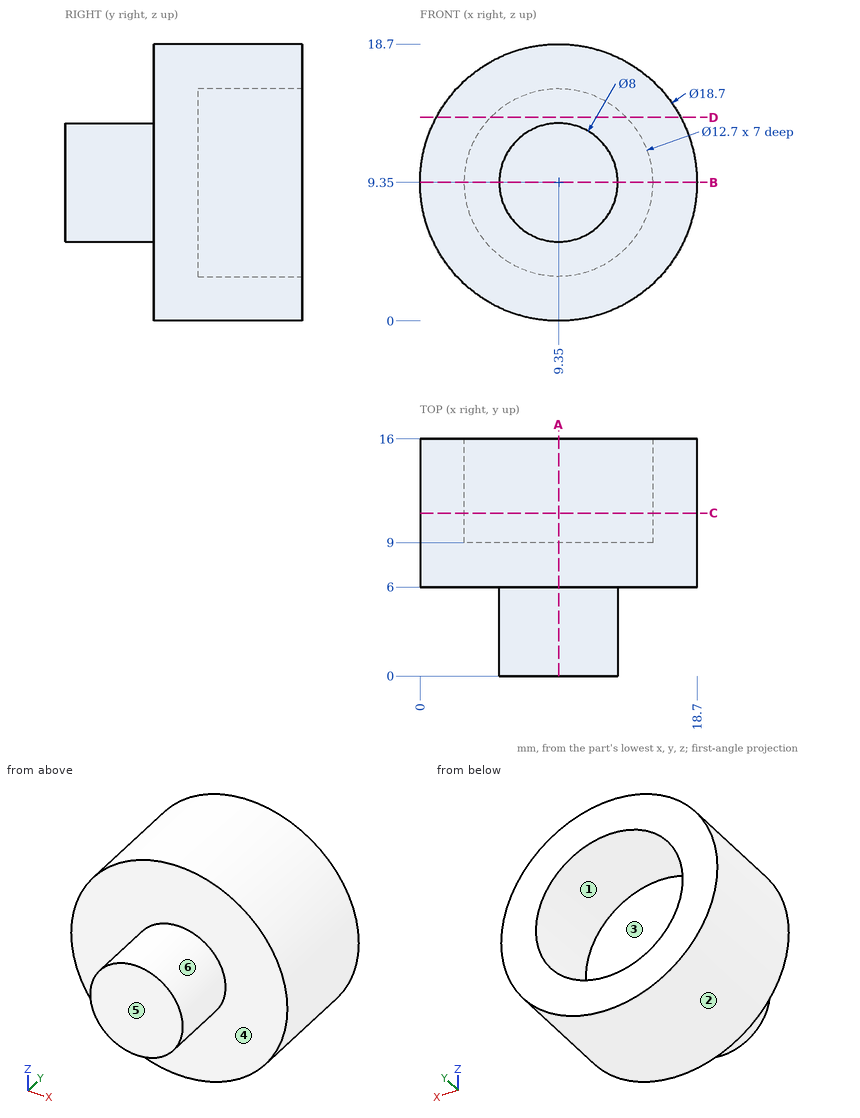
Part print with two shaded views. Sizes in mm from the minimum x, y, z corner. A direction names the side the tool comes from. Round coordinates to 2 decimals unless told otherwise and drop trailing zeros. Write each loop counter-clockwise with the first axis right and the second up, starting at its lowest first coordinate (ties: lowest second). Pieces come first, ordered by that corner, then holes. Notation, with made-up numbers: (31.25, 59.25) -> (36.25, 59.25) arc R21 cw to (36.25, 67.25) -> close; hole circle Ø4 at (84, 38). An arc over 180 degrees is marked (long way). Use one line per item in the form item = value.
Q1. Band-saw the part on D-D, the plane z = 13.75. Write the cut outline in (x, y), then the cut area to 3 significant figures.
Conclusion:
outline = (1.1, 6) -> (17.6, 6) -> (17.6, 16) -> (13.93, 16) -> (13.93, 9) -> (4.77, 9) -> (4.77, 16) -> (1.1, 16) -> close
area = 101 mm²
Q2. Tool access for the marked faces 5 and 6: list every direction of +Z, -Z, +X, -X, +Y, -Y with a clear straight run to the whole face (end or side of a thin tool).
Conclusion:
face_5 = +Z, -Z, +X, -X, -Y
face_6 = -Y
Q3. Drop flat-ended pins along their axis: P1, Ø10, axis at x = 10.5, z = 9, coming from the +Y side; P2, Ø3, axis at x = 3, y = 7.5, coming from the +Z side; P3, Ø10, axis at x = 16, z = 3, coming from the -Y side. Give the stop position or say it passes through.
Conclusion:
P1 = 9
P2 = 17.34
P3 = 6
Q4. Band-saw the part on B-B, the plane z = 9.35. Write the cut outline in (x, y).
Conclusion:
outline = (0, 6) -> (5.35, 6) -> (5.35, 0) -> (13.35, 0) -> (13.35, 6) -> (18.7, 6) -> (18.7, 16) -> (15.7, 16) -> (15.7, 9) -> (3, 9) -> (3, 16) -> (0, 16) -> close
Q5. Two-plate mould, pull along X, no slides. Class the marked faces 1, 2, 3 and 4: released by +X, released by -X, zero draft, split by the parting line, or undercut.
Conclusion:
face_1 = undercut
face_2 = split by the parting line
face_3 = undercut
face_4 = zero draft
Q6. Drill centre lines: L1, parallel to Z at x = 9.35, y = 11.25; L2, parallel to Y at x = 15, z = 6.25. Where is each one in solid material? Low to high.
Conclusion:
L1 = 0 to 3, 15.7 to 18.7
L2 = 6 to 16
Q7. Band-saw the part on A-A, the plane x = 9.35. Write the cut outline in (y, z), then the cut area to 3 significant figures.
Conclusion:
outline = (0, 5.35) -> (6, 5.35) -> (6, 0) -> (16, 0) -> (16, 3) -> (9, 3) -> (9, 15.7) -> (16, 15.7) -> (16, 18.7) -> (6, 18.7) -> (6, 13.35) -> (0, 13.35) -> close
area = 146 mm²
Q8. Band-saw the part on C-C, the plane y = 11. Write the cut outline in (x, z).
Conclusion:
outline = circle Ø18.7 at (9.35, 9.35); hole circle Ø12.7 at (9.35, 9.35)
